Print and shaded views of the part. All mm, measured from the part's lowest x, y and z. Coordinates: 2 decimals unless noted, no trailing zeros. Order: outer loops, then holes, each group sorted by start corner. A loop starts at its lowest first (then second) coordinate and runs counter-clockwise, first axis right, second up. Notation, with made-up numbers: (71, 4.25) -> (82, 4.25) arc R13 cw to (82, 8.25) -> close; hole circle Ø9 at (22, 68). An arc over 180 degrees is marked (long way). Use one line per item in the form item = value. Start each with the question number.
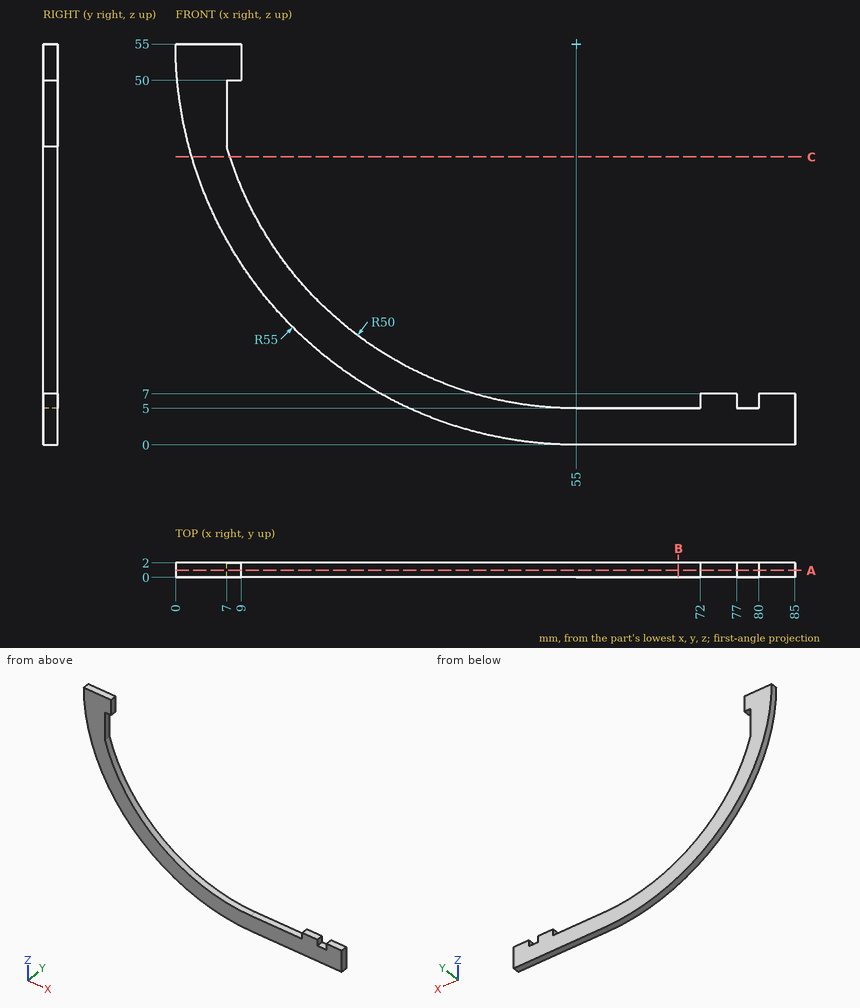
1) Probe L1, parallel to Z at x = 57, y = 1.7; L2, parallel to X at y = 0.45, z = 41.5; L3, parallel to Z at x = 36.5, y = 1.7. List the from-to ranges inside material, lowest first.
2) Cut at C-C on z = 39.5. Give the cut face in (x, y).
3) Cut at B-B on x = 69. Give the cut face in (y, z), then the cut area to 3 significant figures.
4) Drop flat-ended pins along their axis: P1, Ø1, axis at y = 1, z = 5.5, coming from the -X side; P2, Ø1, axis at x = 78, y = 1, coming from the +Z side; P3, Ø1, axis at y = 1.5, z = 31, coming from the -X side. Give the stop position or say it passes through.
5) Cut at A-A on y = 0.95. Give the cut face in (x, z).
Values follow:
q1.L1 = 0 to 5
q1.L2 = 1.68 to 7
q1.L3 = 3.2 to 8.55
q2.outline = (2.23, 0) -> (7.46, 0) -> (7.46, 2) -> (2.23, 2) -> close
q3.outline = (0, 0) -> (2, 0) -> (2, 5) -> (0, 5) -> close
q3.area = 10.0 mm^2
q4.P1 = 30.02
q4.P2 = 5
q4.P3 = 5.27
q5.outline = (0, 55) arc R55 ccw to (55, 0) -> (85, 0) -> (85, 7) -> (80, 7) -> (80, 5) -> (77, 5) -> (77, 7) -> (72, 7) -> (72, 5) -> (55, 5) arc R50 cw to (7, 41) -> (7, 50) -> (9, 50) -> (9, 55) -> close
